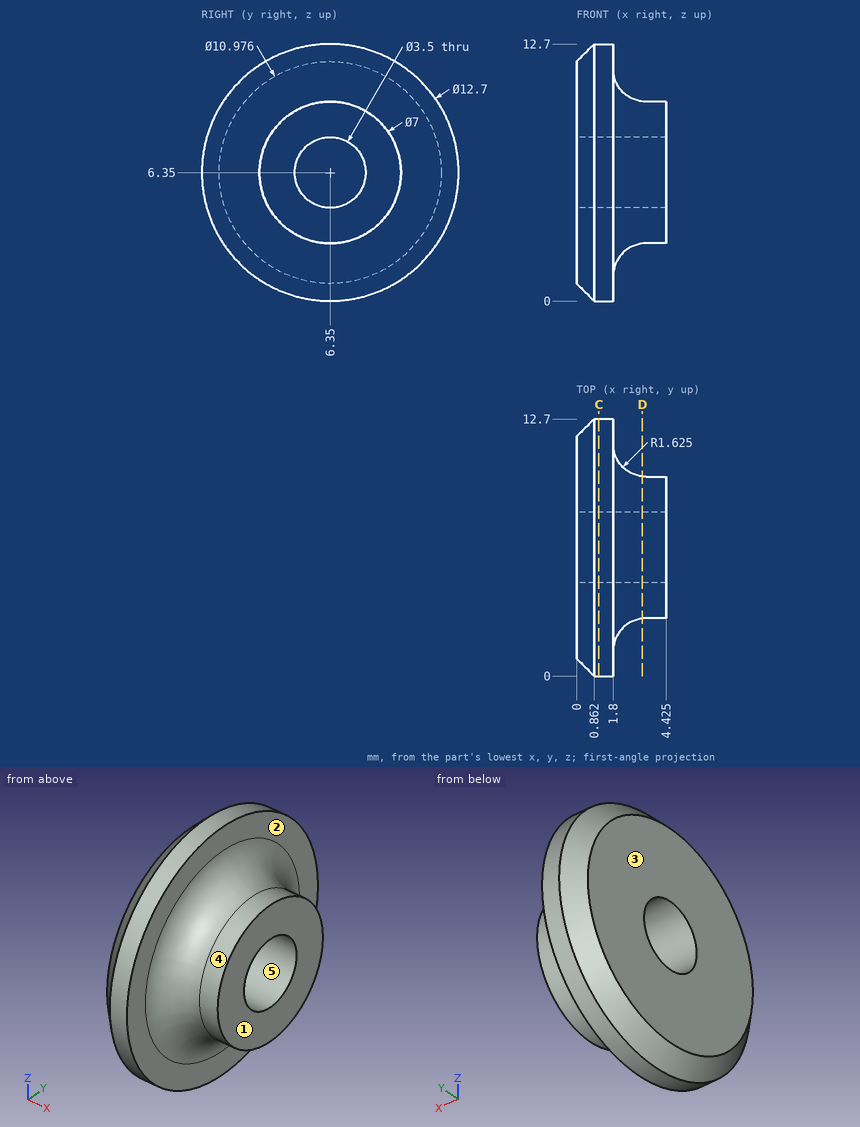
Could you check a few things on this drawing? It's one solid part, dimensions in mm from its lowest x, y, z. A direction names the side the tool comes from. Give positions to 0.01 mm unless a question says otherwise; leave off trailing zeros. Write each loop counter-clockwise with the first axis right and the second up, starting at its lowest first coordinate (ties: lowest second). Pieces come first, ordered by that corner, then holes. Notation, with made-up numbers: (-10, 78) -> (30, 78) arc R25 ccw to (30, 102) -> close; hole circle Ø10 at (54.5, -7). An arc over 180 degrees is marked (long way). Write item = value, one per line.
(1) I need wall thicknesses on probe 1 along Z at (x, y) = (1.5, 6.35); probe 2 along Y at (x, z) = (3.45, 6.35); probe 3 along Y at (x, z) = (2.45, 6.35) (1 decimal). Which ranges of each line are inside material? Lowest first, please. Write a range as from..to.
Worked out:
probe_1 = 0..4.6, 8.1..12.7
probe_2 = 2.85..4.6, 8.1..9.85
probe_3 = 2.5..4.6, 8.1..10.2
(2) Suppose I cut it at D-D on x = 3.25. Write out the boundary of the cut face in (y, z).
Worked out:
outline = circle Ø7.02 at (6.35, 6.35); hole circle Ø3.5 at (6.35, 6.35)
(3) For the marked faces 1 and 2, which set-ups out of +Z, -Z, +X, -X, +Y, -Y let a thin tool reach every point of the face, with its end or its side?
Worked out:
face_1 = +Z, -Z, +X, +Y, -Y
face_2 = +X
(4) I'm going to push flat-ended pins straight in: P1, Ø1, axis at x = 2, y = 9, coming from the +Z side; P2, Ø2, axis at x = 2, y = 3.5, coming from the -Z side; P3, Ø1.5, axis at y = 8.5, z = 11.5, coming from the -X side. Where does each tip first touch, or does it pass through?
Worked out:
P1 = 12.31
P2 = 0.28
P3 = 0
(5) Thinking about a two-plate mould opening in Y: for the marked faces 3, 4 and 5, which applies, released by +Y, released by -Y, zero draft, split by the parting line, or undercut?
Worked out:
face_3 = zero draft
face_4 = split by the parting line
face_5 = undercut
(6) Suppose I cut it at C-C on x = 1.1. Write out the boundary of the cut face in (y, z).
Worked out:
outline = circle Ø12.7 at (6.35, 6.35); hole circle Ø3.5 at (6.35, 6.35)
